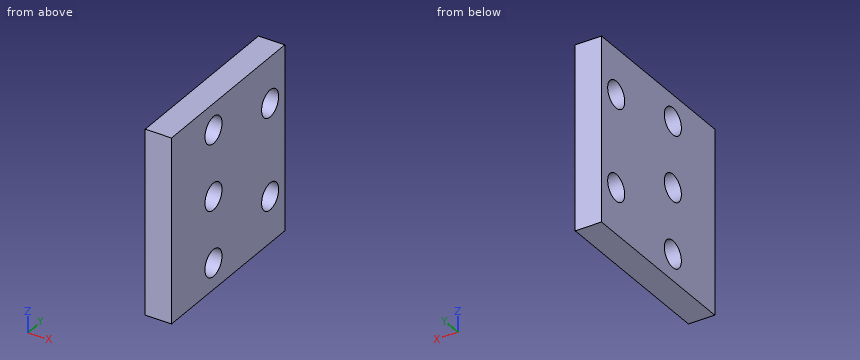
from build123d import *

# Parameters (mm, degrees)
SKETCH1_W           = 35.56
SKETCH1_H           = 34.29
BOSS_EXTRUDE1_DEPTH = 5.08
SKETCH2_R           = 2.5781
CUT_EXTRUDE1_DEPTH  = 26.216776658


with BuildPart() as part:
    # Sketch1 → Boss-Extrude1 (new body)
    with BuildSketch(Plane(origin=(0, 0, 0), x_dir=(0, 0, -1), z_dir=(1, 0, 0))):
        Rectangle(SKETCH1_W, SKETCH1_H)
    extrude(amount=BOSS_EXTRUDE1_DEPTH)

    # Sketch2 → Cut-Extrude1 (cut, through all)
    with BuildSketch(Plane(origin=(5.08, 0, 0), x_dir=(0, 0, -1), z_dir=(1, 0, 0))):
        with Locations((-8.89, 12.7)):
            Circle(SKETCH2_R)
        with Locations((8.89, 12.7)):
            Circle(SKETCH2_R)
        with Locations((-12.7, -4.445)):
            Circle(SKETCH2_R)
        with Locations((0, -4.445)):
            Circle(SKETCH2_R)
        with Locations((12.7, -4.445)):
            Circle(SKETCH2_R)
    extrude(amount=-CUT_EXTRUDE1_DEPTH, mode=Mode.SUBTRACT)


solid = part.part
CAD build for the part. Positions are in the model's coordinates, mm. Give positions to 0.01 mm unless a question says otherwise; leave off trailing zeros. Order: outer loops, then holes, each group sorted by start corner. A loop starts at its lowest first (then second) coordinate and runs counter-clockwise, first axis right, second up. Notation, with made-up numbers: (43, 4.25) -> (92, 4.25) arc R16 ccw to (92, 32.25) -> close; hole circle Ø11 at (36, 50.25). An arc over 180 degrees is marked (long way). Return JSON: item names as keys, results as strings.
Q1. Saw through at A-A (z = 8.89). Write the cut outline in (x, y) (3 decimals).
Working result:
{"outline": "(0, -17.145) -> (5.08, -17.145) -> (5.08, 10.122) -> (0, 10.122) -> close; (0, 15.278) -> (5.08, 15.278) -> (5.08, 17.145) -> (0, 17.145) -> close"}
Q2. Drill centre lines: line 1 (Y direction, x = 2.6, z = -8.89) (3 decimals); line 2 (Z direction, x = 3.8, y = 14.5); line 3 (Z direction, x = 3.85, y = 11). Where is each one in solid material? Low to high.
Working result:
{"line 1": "-17.145 to 10.122, 15.278 to 17.145", "line 2": "-17.78 to -10.74, -7.04 to 7.04, 10.74 to 17.78", "line 3": "-17.78 to -10.83, -6.95 to 6.95, 10.83 to 17.78"}
Q3. Saw through at D-D (y = -4). Write the cut outline in (x, z), then the cut area to 3 significant figures.
Working result:
{"outline": "(0, -17.78) -> (5.08, -17.78) -> (5.08, -15.24) -> (0, -15.24) -> close; (0, -10.16) -> (5.08, -10.16) -> (5.08, -2.54) -> (0, -2.54) -> close; (0, 2.54) -> (5.08, 2.54) -> (5.08, 10.16) -> (0, 10.16) -> close; (0, 15.24) -> (5.08, 15.24) -> (5.08, 17.78) -> (0, 17.78) -> close", "area": "103 mm²"}
Q4. Flat gauge pin, fed straight in: pin 1 (8 mm diameter, centred on y = 12.7, z = 8.89, fed in from -X). Where does the tip first touch, or does it go through?
Working result:
{"pin 1": "x = 0"}
Q5. Saw through at C-C (x = 4.45). Write the cut outline in (y, z) (3 decimals).
Working result:
{"outline": "(-17.145, -17.78) -> (17.145, -17.78) -> (17.145, 17.78) -> (-17.145, 17.78) -> close; hole circle Ø5.156 at (-4.445, -12.7); hole circle Ø5.156 at (-4.445, 0); hole circle Ø5.156 at (-4.445, 12.7); hole circle Ø5.156 at (12.7, -8.89); hole circle Ø5.156 at (12.7, 8.89)"}
Q6. Saw through at B-B (y = 13.5). Write the cut outline in (x, z).
Working result:
{"outline": "(0, -17.78) -> (5.08, -17.78) -> (5.08, -11.34) -> (0, -11.34) -> close; (0, -6.44) -> (5.08, -6.44) -> (5.08, 6.44) -> (0, 6.44) -> close; (0, 11.34) -> (5.08, 11.34) -> (5.08, 17.78) -> (0, 17.78) -> close"}
